Could you check a few things on this drawing? It's one solid part, dimensions in mm from its lowest x, y, z. A direction names the side the tool comes from. Give positions to 0.01 mm unless a question says otherwise; leave off trailing zeros. Loops run counter-clockwise (first coordinate to the right, second up) from the corner with the lowest first, then second, coordinate; pieces in that order, holes last.
Q1. I'm going to push a flat-ended pin straight in: P1, Ø6, axis at x = 13.5, z = 6.5, coming from the +Y side. Where does the tip first touch, or does it pass through?
Q2. Suppose I cut it at A-A (x = 14.25). List the corners of the cut face in (y, z) for me.
Q3. Suppose I cut it at B-B (z = 6.25). List the corners of the cut face in (x, y) for me.
Q4. Thinking about a two-plate mould opening in X: for the marked faces 3, 4 and 5, which applies, pulls with the +X half, pulls with the -X half, needs draft (parallel to the pull), parting line crosses it, or undercut?
Q5. Suppose I cut it at C-C (y = 91). List the corners of the cut face in (x, z) for me, and give its area (3 significant figures).
Q6. For the marked faces 1 and 2, which set-ups out of +Z, -Z, +X, -X, +Y, -Y let a thin tool reach every point of the face, with its end or its side?
Q7. I need wall thicknesses on probe 1 along X at (y, z) = (101, 9). Which ranges of the line are inside material? Lowest first, please.
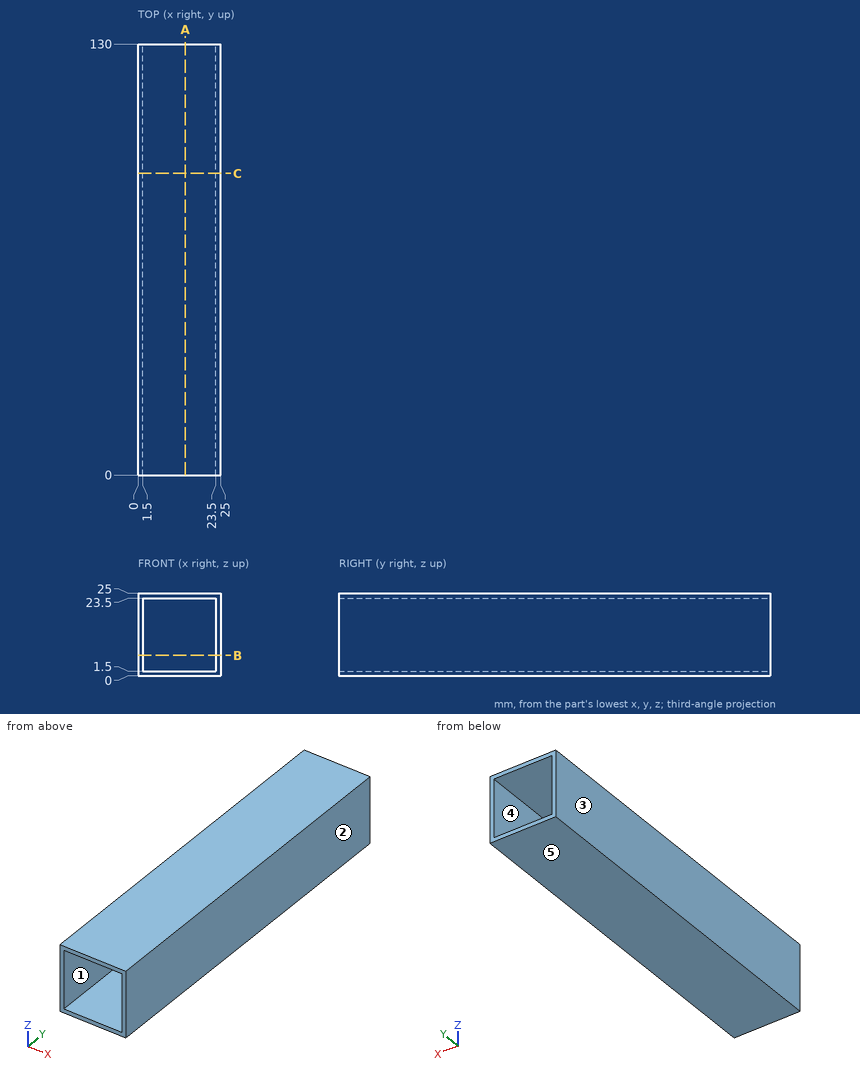
Solutions:
1. P1: passes through
2. outline: (0, 0) - (130, 0) - (130, 1.5) - (0, 1.5) - close; (0, 23.5) - (130, 23.5) - (130, 25) - (0, 25) - close
3. outline: (0, 0) - (1.5, 0) - (1.5, 130) - (0, 130) - close; (23.5, 0) - (25, 0) - (25, 130) - (23.5, 130) - close
4. face 3: pulls with the -X half
4. face 4: undercut
4. face 5: needs draft
5. outline: (0, 0) - (25, 0) - (25, 25) - (0, 25) - close; hole (1.5, 1.5) - (23.5, 1.5) - (23.5, 23.5) - (1.5, 23.5) - close
5. area: 141 mm2
6. face 1: +Y, -Y
6. face 2: +Z, -Z, +X, +Y, -Y
7. probe 1: x = 0 to 1.5, 23.5 to 25
